```python
from build123d import *

# Parameters (mm, degrees)
SKETCH1_R                = 6.35
BOSS_EXTRUDE1_DEPTH      = 300
SKETCH2_W                = 3
SKETCH2_H                = 101.6
BOSS_EXTRUDE2_DEPTH      = 300
CIRPATTERN1_COUNT        = 9
SKETCH9_R                = 60.024928634
SKETCH9_R_2              = 25.4
CUT_EXTRUDE1_DEPTH       = 317.2
SKETCH11_W               = 209.953471272
SKETCH11_H               = 400
CUT_EXTRUDE2_DEPTH       = 158.6
SKETCH13_R               = 5
BOSS_EXTRUDE3_DEPTH      = 260
BOSS_EXTRUDE3_DEPTH_BACK = 20
SKETCH14_R               = 26
BOSS_EXTRUDE4_DEPTH      = 20
SKETCH15_R               = 26
BOSS_EXTRUDE5_DEPTH      = 20


with BuildPart() as part:
    # Sketch1 → Boss-Extrude1 (new body)
    with BuildSketch(Plane.XY):
        Circle(SKETCH1_R)
    extrude(amount=BOSS_EXTRUDE1_DEPTH)

    # Sketch2 → Boss-Extrude2 (add, through all)
    with BuildSketch(Plane.XY.offset(300)):
        Rectangle(SKETCH2_W, SKETCH2_H)
    boss_extrude2 = extrude(amount=-BOSS_EXTRUDE2_DEPTH)

    # CirPattern1: Boss-Extrude2 ×9 about axis
    cirpattern1_axis = Axis((0, 0, 0), (0, 0, 1))
    for i in range(1, CIRPATTERN1_COUNT):
        add(boss_extrude2.rotate(cirpattern1_axis, i * 360 / CIRPATTERN1_COUNT))

    # Sketch9 → Cut-Extrude1 (cut)
    with BuildSketch(Plane.XY.offset(300)):
        Circle(SKETCH9_R)
        Circle(SKETCH9_R_2, mode=Mode.SUBTRACT)
    extrude(amount=-CUT_EXTRUDE1_DEPTH, mode=Mode.SUBTRACT)

    # Sketch11 → Cut-Extrude2 (cut, symmetric)
    with BuildSketch(Plane(origin=(0, 0, 0), x_dir=(1, 0, 0), z_dir=(0, 1, 0))):
        with Locations((-1.595391119, -400)):
            Rectangle(SKETCH11_W, SKETCH11_H)
    extrude(amount=CUT_EXTRUDE2_DEPTH, both=True, mode=Mode.SUBTRACT)

    # Sketch13 → Boss-Extrude3 (add, two sides)
    with BuildSketch(Plane.XY) as boss_extrude3_sk:
        Circle(SKETCH13_R)
    extrude(amount=BOSS_EXTRUDE3_DEPTH)
    extrude(boss_extrude3_sk.sketch, amount=-BOSS_EXTRUDE3_DEPTH_BACK)

    # Sketch14 → Boss-Extrude4 (add)
    with BuildSketch(Plane(origin=(0, 0, 0), x_dir=(-1, 0, 0), z_dir=(0, 0, -1))):
        Circle(SKETCH14_R)
    extrude(amount=-BOSS_EXTRUDE4_DEPTH)

    # Sketch15 → Boss-Extrude5 (add)
    with BuildSketch(Plane.XY.offset(200)):
        Circle(SKETCH15_R)
    extrude(amount=-BOSS_EXTRUDE5_DEPTH)


solid = part.part
```
Check sheet for the modelled part. Datum: model origin and axes. Units: mm. A direction names the side the tool comes from. Coordinates: 2 decimals unless noted, no trailing zeros. Order: outer loops, then holes, each group sorted by start corner. A loop starts at its lowest first (then second) coordinate and runs counter-clockwise, first axis right, second up. Notation, with made-up numbers: (-10.5, 14.25) -> (44.5, 14.25) arc R13 ccw to (44.5, 18.25) -> close; hole circle Ø10 at (49, -16). An arc over 180 degrees is marked (long way). Write each question's results on one line, items separated by ' | '. Start each with the question number.
1) Section check A-A (z = 204.5). Enter the section's corners in (x, y), and give its area (3 significant figures).
2) Depth check by flat-ended pin: pin 1 (6 mm diameter, centred on x = -17, z = 180, fed in from +Y); pin 2 (1 mm diameter, centred on x = -19.5, y = 9, fed in from +Z); pin 3 (3 mm diameter, centred on x = 12, y = -2.5, fed in from -Z). Enter the tip coordinate at first touch or a pass-through.
3) Draft check along Y on faces 1 (the face through (-5.4, 0.4, 0)), 2 (the face through (16.297, 4.397, 101.12)), 3 (the face through (20.633, -15.821, 9.86)), 4 (the face through (16.53, -4.438, 101.12)). Enter one of: pulls with the +Y half, pulls with the -Y half, needs draft (parallel to the pull), parting line crosses it, or undercut.
4) Set-up check for faces 5 (the face through (0, 0, -20)), 6 (the face through (-15.3, -7.1, 101.1)): record each of +Z, -Z, +X, -X, +Y, -Y from which the full face is reachable in a straight line by a thin tool's end or side.
5) Material ranges on line 1 along Z through (x, y) = (2, 15); line 2 along Y through (x, z) = (-16, 21.5); line 3 along Y through (x, z) = (15, 158), recorded low to high.
Checked values:
1) outline: circle Ø10 at (0, 0) | area: 78.5 mm²
2) pin 1: y = 21.91 | pin 2: z = 200 | pin 3: z = 0
3) face 1: needs draft | face 2: undercut | face 3: parting line crosses it | face 4: undercut
4) face 5: -Z, +X, -X, +Y, -Y | face 6: none
5) line 1: 0 to 20, 180 to 200 | line 2: -19.73 to -16.73, -10.97 to -7.51, -4.34 to -1.3, 1.3 to 4.34, 7.51 to 10.97, 16.73 to 19.73 | line 3: -20.21 to -15.54, -10.39 to -6.93, -4.17 to -1.12, 1.12 to 4.17, 6.93 to 10.39, 15.54 to 20.21
